Verification items for the finished model (mm, model axes). A direction names the side the tool comes from. Coordinates: 2 decimals unless noted, no trailing zeros. Write each loop counter-clockwise with the first axis right and the second up, starting at its lowest first coordinate (ties: lowest second). Pieces come first, ordered by that corner, then holes. Notation, with made-up numbers: (60.5, 37) -> (92.5, 37) arc R24 cw to (92.5, 73) -> close; hole circle Ø11 at (-14, -34). An arc over 180 degrees is marked (long way). Write item = value, one per line. Start each with the question number.
(1) Section check A-A (x = -161). Record the cut outline in (y, z), plus the area to 3 significant figures.
(2) Section check C-C (x = -133). Record the cut outline in (y, z), plus the area to 3 significant figures.
(3) Set-up check for faces 4 (the face through (-122.139, -182.694, 2.958)), 5 (the face through (-172.563, -193, 3)), 6 (the face through (-172.563, -154, 3)): record each of +Z, -Z, +X, -X, +Y, -Y from which the full face is reachable in a straight line by a thin tool's end or side.
(4) Gauge pin test, flat ends, axial feed: pin 1 Ø10 at (x, y) = (-129.5, -170.5) entering from +Z; pin 2 Ø1.3 at (x, z) = (-175, 3.5) entering from -Y; pin 3 Ø1.4 at (y, z) = (-170.5, 4) entering from -X. Record the tip position at first contact, or that the pin passes through.
(5) Material ranges on probe 1 along Y at (x, z) = (-115.5, 3.05); probe 2 along Y at (x, z) = (-168, 5.8); probe 3 along Y at (x, z) = (-165, 2.6), recorded low to high. Write a range as [from, to].
(6) Mould release check, pull along X, two halves, no side actions. Record for faces 1 (the face through (-162.163, -177, 3)), 2 (the face through (-151, -173, 6)), 3 (the face through (-109.53, -153.09, 2.96)): released by +X, released by -X, zero draft, split by the parting line, or undercut.
(7) Section check B-B (z = 4.95). State how many separate pieces and enclosed holes the cut face has, plus the area to 3 significant figures.
```python
from build123d import *

# Parameters (mm, degrees)
BOSS_EXTRUDE1_DEPTH = 6


with BuildPart() as part:
    # Sketch1 → Boss-Extrude1 (new body)
    with BuildSketch(Plane.XY):
        Polygon((-107.062987014, -155.556624264), (-112.062985414, -150.556625864), (-172.562973402, -150.556625864), (-172.562973402, -157.335700029), (-176.912971293, -157.335700029), (-177.430609383, -157.403848376), (-177.912971293, -157.603649221), (-178.327184855, -157.921486467), (-178.6450221, -158.335700029), (-178.844822945, -158.818061939), (-178.912971293, -159.335700029), (-178.912971293, -164.135695994), (-178.844822945, -164.653334084), (-178.6450221, -165.135695994), (-178.327184855, -165.549909556), (-177.912971293, -165.867746802), (-177.430609383, -166.067547647), (-176.912971293, -166.135695994), (-172.562973402, -166.135695994), (-172.562973402, -171.435688001), (-167.26297458, -171.435688001), (-167.26297458, -169.635689769), (-162.162976815, -169.635689769), (-162.162976815, -171.435688001), (-158.212977143, -171.435688001), (-158.212977143, -175.835692673), (-162.162976966, -175.835692673), (-162.162976966, -177.635690904), (-167.26297473, -177.635690904), (-167.26297473, -175.835692673), (-172.562973552, -175.835692673), (-172.562973552, -181.135689927), (-176.912971443, -181.135689927), (-177.430609533, -181.203838275), (-177.912971443, -181.40363912), (-178.327185006, -181.721476365), (-178.645022251, -182.135689927), (-178.844823096, -182.618051837), (-178.912971443, -183.135689927), (-178.912971443, -187.93568437), (-178.844823096, -188.45332246), (-178.645022251, -188.93568437), (-178.327185006, -189.349897932), (-177.912971443, -189.667735177), (-177.430609533, -189.867536022), (-176.912971443, -189.93568437), (-172.562973552, -189.93568437), (-172.562973552, -195.556608264), (-112.062985371, -195.556608264), (-107.062987014, -190.556608264), align=None)
        Polygon((-150.762975594, -156.535695809), (-151.177085934, -156.590214469), (-151.562975338, -156.750055094), (-151.894346082, -157.004324809), (-152.148615797, -157.335695553), (-152.308456422, -157.721584957), (-152.362975082, -158.135695297), (-152.308456422, -158.549805636), (-152.148615797, -158.935695041), (-151.894346082, -159.267065785), (-151.562975338, -159.521335499), (-151.177085934, -159.681176124), (-150.762975594, -159.735694785), (-144.562976618, -159.735694785), (-144.148866278, -159.681176124), (-143.762976874, -159.521335499), (-143.43160613, -159.267065785), (-143.177336415, -158.935695041), (-143.017495791, -158.549805636), (-142.96297713, -158.135695297), (-143.017495791, -157.721584957), (-143.177336415, -157.335695553), (-143.43160613, -157.004324809), (-143.762976874, -156.750055094), (-144.148866278, -156.590214469), (-144.562976618, -156.535695809), align=None, mode=Mode.SUBTRACT)
        Polygon((-143.431606507, -188.004315269), (-143.762977251, -187.750045554), (-144.148866655, -187.590204929), (-144.562976995, -187.535686269), (-150.762975971, -187.535686269), (-151.17708631, -187.590204929), (-151.562975715, -187.750045554), (-151.894346459, -188.004315269), (-152.148616173, -188.335686013), (-152.308456798, -188.721575417), (-152.362975459, -189.135685757), (-152.308456798, -189.549796096), (-152.148616173, -189.935685501), (-151.894346459, -190.267056245), (-151.562975715, -190.521325959), (-151.17708631, -190.681166584), (-150.762975971, -190.735685245), (-144.562976995, -190.735685245), (-144.148866655, -190.681166584), (-143.762977251, -190.521325959), (-143.431606507, -190.267056245), (-143.177336792, -189.935685501), (-143.017496167, -189.549796096), (-142.962977507, -189.135685757), (-143.017496167, -188.721575417), (-143.177336792, -188.335686013), align=None, mode=Mode.SUBTRACT)
        Polygon((-121.362985002, -189.135685377), (-121.308466342, -189.549795716), (-121.148625717, -189.935685121), (-120.894356002, -190.267055865), (-120.562985258, -190.521325579), (-120.177095854, -190.681166204), (-119.762985514, -190.735684865), (-113.562986538, -190.735684865), (-113.148876198, -190.681166204), (-112.762986794, -190.521325579), (-112.43161605, -190.267055865), (-112.177346335, -189.935685121), (-112.017505711, -189.549795716), (-111.96298705, -189.135685377), (-112.017505711, -188.721575037), (-112.177346335, -188.335685633), (-112.43161605, -188.004314889), (-112.762986794, -187.750045174), (-113.148876198, -187.590204549), (-113.562986538, -187.535685889), (-119.762985514, -187.535685889), (-120.177095854, -187.590204549), (-120.562985258, -187.750045174), (-120.894356002, -188.004314889), (-121.148625717, -188.335685633), (-121.308466342, -188.721575037), align=None, mode=Mode.SUBTRACT)
        Polygon((-119.762985514, -156.535695809), (-113.562986538, -156.535695809), (-113.148876198, -156.590214469), (-112.762986794, -156.750055094), (-112.43161605, -157.004324809), (-112.177346335, -157.335695553), (-112.017505711, -157.721584957), (-111.96298705, -158.135695297), (-112.017505711, -158.549805636), (-112.177346335, -158.935695041), (-112.43161605, -159.267065785), (-112.762986794, -159.521335499), (-113.148876198, -159.681176124), (-113.562986538, -159.735694785), (-119.762985514, -159.735694785), (-120.177095854, -159.681176124), (-120.562985258, -159.521335499), (-120.894356002, -159.267065785), (-121.148625717, -158.935695041), (-121.308466342, -158.549805636), (-121.362985002, -158.135695297), (-121.308466342, -157.721584957), (-121.148625717, -157.335695553), (-120.894356002, -157.004324809), (-120.562985258, -156.750055094), (-120.177095854, -156.590214469), align=None, mode=Mode.SUBTRACT)
        Polygon((-126.086563512, -184.743833784), (-123.312983418, -183.594979293), (-120.931256197, -181.767415718), (-119.103692622, -179.385688497), (-117.95483813, -176.612108403), (-117.562985258, -173.635690337), (-117.95483813, -170.65927227), (-119.103692622, -167.885692177), (-120.931256197, -165.503964955), (-123.312983418, -163.67640138), (-126.086563512, -162.527546889), (-129.062981578, -162.135694017), (-135.262980554, -162.135694017), (-138.23939862, -162.527546889), (-141.012978714, -163.67640138), (-143.394705936, -165.503964955), (-145.222269511, -167.885692177), (-146.371124002, -170.65927227), (-146.762976874, -173.635690337), (-146.371124002, -176.612108403), (-145.222269511, -179.385688497), (-143.394705936, -181.767415718), (-141.012978714, -183.594979293), (-138.23939862, -184.743833784), (-135.262980554, -185.135686657), (-129.062981578, -185.135686657), align=None, mode=Mode.SUBTRACT)
    extrude(amount=BOSS_EXTRUDE1_DEPTH)


solid = part.part
```
Response:
q1.outline = (-195.56, 0) -> (-175.84, 0) -> (-175.84, 6) -> (-195.56, 6) -> close; (-171.44, 0) -> (-150.56, 0) -> (-150.56, 6) -> (-171.44, 6) -> close
q1.area = 244 mm2
q2.outline = (-195.56, 0) -> (-185.14, 0) -> (-185.14, 6) -> (-195.56, 6) -> close; (-162.14, 0) -> (-150.56, 0) -> (-150.56, 6) -> (-162.14, 6) -> close
q2.area = 132 mm2
q3.face_4 = +Z, -Z
q3.face_5 = +Z, -Z, -X, -Y
q3.face_6 = +Z, -Z, -X, +Y
q4.pin_1 = through
q4.pin_2 = -189.94
q4.pin_3 = -172.56
q5.probe_1 = [-195.56, -190.74], [-187.54, -159.74], [-156.54, -150.56]
q5.probe_2 = [-195.56, -175.84], [-171.44, -150.56]
q5.probe_3 = [-195.56, -177.64], [-169.64, -150.56]
q6.face_1 = undercut
q6.face_2 = zero draft
q6.face_3 = released by +X
q7.separate_pieces = 1
q7.enclosed_holes = 5
q7.area = 2,280 mm2
